Autodesk Inventor part; units mm, degrees
ref_plane "YZ Plane" through (0, 0, 0) normal (1, 0, 0) x (0, 1, 0)
ref_plane "XZ Plane" through (0, 0, 0) normal (0, 1, 0) x (-1, 0, 0)
ref_plane "XY Plane" through (0, 0, 0) normal (0, 0, 1) x (1, 0, 0)
sketch "Esquisse1" plane through (0, 0, 0) normal (0, 0, 1) x (1, 0, 0)
  line L0 (0, 0) -> (51.5, 0)
  line L1 (51.5, 0) -> (51.5, -75)
  line L2 (51.5, -75) -> (0, -75)
  line L3 (0, -75) -> (0, 0)
  dimension "d0" = 51.5
  dimension "d1" = 75
extrude "Extrusion1" add sketch "Esquisse1" along normal blind 5
sketch "Esquisse2" plane through (0, 0, 5) normal (0, 0, 1) x (1, 0, 0)
  line L0 (0, 0) -> (51.5, 0)
  line L1 (51.5, 0) -> (51.5, -25)
  line L2 (51.5, -25) -> (0, -25)
  line L3 (0, -25) -> (0, 0)
  dimension "d4" = 25
extrude "Extrusion2" cut sketch "Esquisse2" against normal blind 2.5
sketch "Esquisse3" plane through (0, 0, 2.5) normal (0, 0, 1) x (1, 0, 0)
  circle A0 centre (10, -12.5) radius 2.6
  circle A1 centre (41.5, -12.5) radius 2.6
  line L0 (0, 0) -> (51.5, 0)
  line L1 (0, -25) -> (0, 0)
  line L2 (51.5, 0) -> (51.5, -25)
  dimension "d7" = 5.2
  dimension "d8" = 5.2
  dimension "d9" = 12.5
  dimension "d10" = 10
  dimension "d11" = 12.5
  dimension "d12" = 10
extrude "Extrusion3" cut sketch "Esquisse3" against normal blind 2.5
sketch "Esquisse4" plane through (0, 0, 5) normal (0, 0, 1) x (1, 0, 0)
  line L0 (0, -75) -> (51.5, -75)
  line L1 (51.5, -75) -> (51.5, -70)
  line L2 (51.5, -70) -> (0, -70)
  line L3 (0, -70) -> (0, -75)
  dimension "d15" = 5
extrude "Extrusion4" add sketch "Esquisse4" along normal blind 70
sketch "Esquisse6" plane through (0, -75, 0) normal (0, -1, 0) x (1, 0, 0)
  line L0 (51.5, 5) -> (51.5, 75)
  line L1 (51.5, 75) -> (0, 75)
  line L2 (0, 75) -> (0, 80)
  line L3 (0, 80) -> (51.5, 80)
  line L4 (51.5, 80) -> (51.5, 75)
  point P0 (0, 0)
  dimension "d19" = 5
extrude "Extrusion5" add sketch "Esquisse6" against normal blind 75
sketch "Esquisse7" plane through (51.5, -70, 75) normal (0, 0, -1) x (-1, 0, 0)
  line L0 (0, 70) -> (51.5, 70)
  line L1 (0, 70) -> (51.5, 70)
  line L2 (51.5, 70) -> (51.5, 45)
  line L3 (51.5, 45) -> (0, 45)
  line L4 (0, 45) -> (0, 70)
  dimension "d22" = 25
extrude "Extrusion6" cut sketch "Esquisse7" against normal blind 2.5
sketch "Esquisse8" plane through (51.5, -70, 77.5) normal (0, 0, -1) x (-1, 0, 0)
  circle A0 centre (10, 57.5) radius 2.6
  circle A1 centre (41.5, 57.5) radius 2.6
  line L0 (0, 45) -> (0, 70)
  line L1 (51.5, 70) -> (51.5, 45)
  line L2 (0, 70) -> (51.5, 70)
  dimension "d25" = 5.2
  dimension "d26" = 5.2
  dimension "d27" = 10
  dimension "d28" = 10
  dimension "d29" = 12.5
  dimension "d30" = 12.5
extrude "Extrusion7" cut sketch "Esquisse8" against normal blind 2.5
sketch "Esquisse9" plane through (0, -75, 0) normal (0, -1, 0) x (1, 0, 0)
  line L0 (0, 80) -> (51.5, 80) construction
  line L1 (51.5, 0) -> (51.5, 2.5) construction
  line L2 (0, 80) -> (51.5, 0) construction
  line L3 (51.5, 80) -> (0, 0) construction
  circle A0 centre (25.75, 40) radius 4
  dimension "d33" = 8
extrude "Extrusion8" cut sketch "Esquisse9" against normal blind 5
sketch "Esquisse10" plane through (0, 0, 5) normal (0, 0, 1) x (1, 0, 0)
  line L0 (0, -70) -> (51.5, -70) construction
  line L1 (51.5, -25) -> (0, -25) construction
  line L2 (0, -70) -> (51.5, -25) construction
  line L3 (51.5, -70) -> (51.5, -25) construction
  line L4 (0, -25) -> (0, -70) construction
  line L5 (51.5, -70) -> (0, -25) construction
  circle A0 centre (25.75, -47.5) radius 5
  point P0 (0, 0)
  dimension "d36" = 10
extrude "Extrusion9" add sketch "Esquisse10" along normal blind 70
properties part number "Forearm2 v2" material "Plastique ABS"
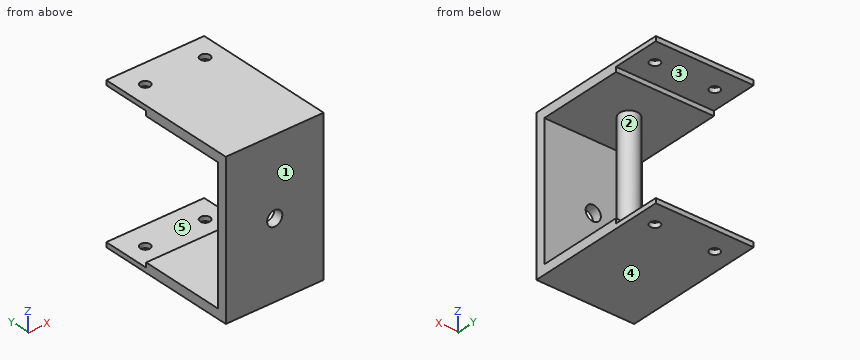
Geometry: final body of the model. Coordinates: model frame, mm. Face numbers are marked on the shaded views. A direction names the side the tool comes from. Give positions to 0.01 mm unless a question says otherwise; leave off trailing zeros. Order: outer loops, then holes, each group sorted by start corner. A loop starts at its lowest first (then second) coordinate and runs counter-clockwise, first axis right, second up. Notation, with made-up numbers: (-1, 23) - (15, 23) arc R12 cw to (15, 43) - close; hole circle Ø11 at (-12, -15.5). An arc over 180 degrees is marked (long way). Use CSV: the item, a comma, the result in double quotes.
1. Section query D-D (z = 65.5). Output: boundary loops of the cut face in (x, y), plus the area to 3 significant figures.
Answers below:
outline,"(0, -75) - (51.5, -75) - (51.5, -70) - (0, -70) - close; circle Ø10 at (25.75, -47.5)"
area,"336 mm2"
2. Mould query, pull axis Y, two halves, no side actions, for the marked faces 1, 2 and 3. Classes: +Y half, -Y half, draft (parallel to the pull), parting line (faces both ways), or undercut.
Answers below:
face 1,"-Y half"
face 2,"undercut"
face 3,"draft"
3. Section query C-C (y = -12.5). Output: boundary loops of the cut face in (x, z), plus the area to 4 significant figures.
Answers below:
outline,"(0, 0) - (7.4, 0) - (7.4, 2.5) - (0, 2.5) - close; (0, 77.5) - (7.4, 77.5) - (7.4, 80) - (0, 80) - close; (12.6, 0) - (38.9, 0) - (38.9, 2.5) - (12.6, 2.5) - close; (12.6, 77.5) - (38.9, 77.5) - (38.9, 80) - (12.6, 80) - close; (44.1, 0) - (51.5, 0) - (51.5, 2.5) - (44.1, 2.5) - close; (44.1, 77.5) - (51.5, 77.5) - (51.5, 80) - (44.1, 80) - close"
area,"205.5 mm2"
4. Contact query for flat-ended pins moving along their axis: pin 1 (13 mm diameter, centred on x = 25.75, z = 40, fed in from -Y); pin 2 (8 mm diameter, centred on x = 38, z = 50.5, fed in from +Y); pin 3 (0.8 mm diameter, centred on x = 19, z = 4, fed in from +Y). Output: stop coordinate, or through.
Answers below:
pin 1,"y = -75"
pin 2,"y = -70"
pin 3,"y = -25"
5. Access query for the marked faces 4 and 5. Directions: +Z, -Z, +X, -X, +Y, -Y. A direction counts if a zero-diameter tool reaches every point of the face in a straight line with its end or side. Return the directions, or none.
Answers below:
face 4,"-Z, +X, -X, +Y, -Y"
face 5,"+X, -X, +Y"
6. Material intervals for line 1 along Z through (x, y) = (38, -43); line 2 along Z through (x, y) = (12.5, -17.5); line 3 along Y through (x, z) = (41.5, 1.8), sorted ascending. Write a range as from..to.
Answers below:
line 1,"0..5, 75..80"
line 2,"0..2.5, 77.5..80"
line 3,"-75..-15.1, -9.9..0"
7. Section query A-A (x = 41.5). Output: boundary loops of the cut face in (y, z).
Answers below:
outline,"(-75, 0) - (-15.1, 0) - (-15.1, 2.5) - (-25, 2.5) - (-25, 5) - (-70, 5) - (-70, 75) - (-25, 75) - (-25, 77.5) - (-15.1, 77.5) - (-15.1, 80) - (-75, 80) - close; (-9.9, 0) - (0, 0) - (0, 2.5) - (-9.9, 2.5) - close; (-9.9, 77.5) - (0, 77.5) - (0, 80) - (-9.9, 80) - close"
8. Section query B-B (y = -20). Output: boundary loops of the cut face in (x, z), plus the area to 4 significant figures.
Answers below:
outline,"(0, 0) - (51.5, 0) - (51.5, 2.5) - (0, 2.5) - close; (0, 77.5) - (51.5, 77.5) - (51.5, 80) - (0, 80) - close"
area,"257.5 mm2"
